Drawing for the job (mm, zero at the part's lowest x, y, z). A direction names the side the tool comes from. Give positions to 0.01 mm unless a question says otherwise; leave off trailing zeros. Write each loop counter-clockwise with the first axis right and the second up, starting at its lowest first coordinate (ties: lowest second). Pieces come first, ordered by that corner, then holes.
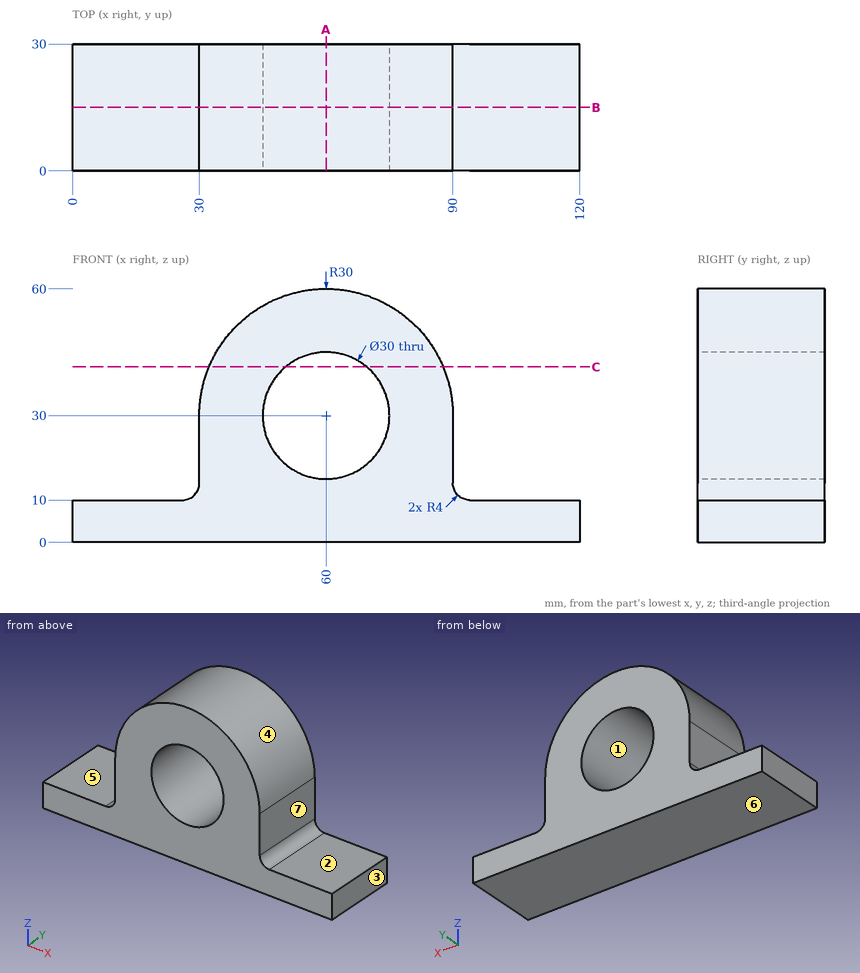
1. Slice it at C-C, the plane z = 41.5. Write the cut outline in (x, y), and give its area (3 significant figures).
Calculated:
outline: (32.29, 0) - (50.37, 0) - (50.37, 30) - (32.29, 30) - close; (69.63, 0) - (87.71, 0) - (87.71, 30) - (69.63, 30) - close
area: 1,080 mm2
2. Slice it at B-B, the plane y = 15. Write the cut outline in (x, z).
Calculated:
outline: (0, 0) - (120, 0) - (120, 10) - (94, 10) arc R4 cw to (90, 14) - (90, 30) arc R30 ccw to (30, 30) - (30, 14) arc R4 cw to (26, 10) - (0, 10) - close; hole circle Ø30 at (60, 30)
3. Which spindle directions (+Z, -Z, +X, -X, +Y, -Y) get a long thin tool onto all of the face, cutting with end or side? Do the marked faces 5, 6 and 7. Say none if no direction does.
Calculated:
face 5: +Z, -X, +Y, -Y
face 6: -Z, +X, -X, +Y, -Y
face 7: +Z, +X, +Y, -Y
4. Probe probe 1 along Z at (x, y) = (60, 18.5); probe 2 along Z at (x, y) = (24, 8.5); probe 3 along X at (y, z) = (8, 17.5). List the from-to ranges inside material, lowest first.
Calculated:
probe 1: z = 0 to 15, 45 to 60
probe 2: z = 0 to 10
probe 3: x = 30 to 51.71, 68.29 to 90
5. Pull direction X, two halves, no side cores. Call the marked faces 1, 2, 3 and 4: +X half, -X half, draft (parallel to the pull), parting line (faces both ways), or undercut.
Calculated:
face 1: undercut
face 2: draft
face 3: +X half
face 4: parting line
6. Pin check, flat tips, straight feed: P1, Ø13, axis at x = 103.5, y = 16.5, coming from the +Z side; P2, Ø4, axis at y = 14.5, z = 21, coming from the +X side; P3, Ø8, axis at y = 15, z = 46, coming from the +X side; P4, Ø8, axis at x = 80.5, y = 15.5, coming from the -Z side. Stop position of each tip, or through.
Calculated:
P1: stops at z = 10
P2: stops at x = 90
P3: stops at x = 87.5
P4: stops at z = 0
7. Slice it at A-A, the plane x = 60. Write the cut outline in (y, z), and give its area (3 significant figures).
Calculated:
outline: (0, 0) - (30, 0) - (30, 15) - (0, 15) - close; (0, 45) - (30, 45) - (30, 60) - (0, 60) - close
area: 900 mm2
